```python
from build123d import *

# Parameters (mm, degrees)
SKETCH1_W           = 44
SKETCH1_H           = 44
BOSS_EXTRUDE1_DEPTH = 3
SKETCH2_W           = 21
SKETCH2_H           = 16
BOSS_EXTRUDE2_DEPTH = 12
SKETCH3_W           = 15
SKETCH3_H           = 10
CUT_EXTRUDE1_DEPTH  = 12
CUT_EXTRUDE2_REACH  = 66.008
FILLET1_R           = 3.175


with BuildPart() as part:
    # Sketch1 → Boss-Extrude1 (new body)
    with BuildSketch(Plane(origin=(0, 0, 0), x_dir=(1, 0, 0), z_dir=(0, 1, 0))):
        with Locations((22, 22)):
            Rectangle(SKETCH1_W, SKETCH1_H)
    extrude(amount=BOSS_EXTRUDE1_DEPTH)

    # Sketch2 → Boss-Extrude2 (add)
    with BuildSketch(Plane(origin=(0, 3, 0), x_dir=(1, 0, 0), z_dir=(0, 1, 0))):
        with Locations((22, 22)):
            Rectangle(SKETCH2_W, SKETCH2_H)
    extrude(amount=BOSS_EXTRUDE2_DEPTH)

    # Sketch3 → Cut-Extrude1 (cut)
    with BuildSketch(Plane.XZ):
        with Locations((22, -22)):
            Rectangle(SKETCH3_W, SKETCH3_H)
    extrude(amount=-CUT_EXTRUDE1_DEPTH, mode=Mode.SUBTRACT)

    # Sketch4 → Cut-Extrude2 (cut, up to next)
    with BuildSketch(Plane(origin=(0, 15, 0), x_dir=(1, 0, 0), z_dir=(0, 1, 0)), mode=Mode.PRIVATE) as cut_extrude2_sk1:
        with BuildLine():
            Line((19.05, 23.2), (24.95, 23.2))
            ThreePointArc((24.95, 23.2), (26.15, 22), (24.95, 20.8))
            Line((24.95, 20.8), (19.05, 20.8))
            ThreePointArc((19.05, 20.8), (17.85, 22), (19.05, 23.2))
        make_face()
    cut_extrude2_tool1 = extrude(cut_extrude2_sk1.sketch, amount=-CUT_EXTRUDE2_REACH, mode=Mode.PRIVATE) & part.part
    add(cut_extrude2_tool1.solids().sort_by_distance((22, 15, -22))[0], mode=Mode.SUBTRACT)

    # Fillet1
    fillet1_edges = [part.edges().sort_by_distance(p)[0] for p in [
        (0, 1.5, -44),
        (44, 1.5, -44),
        (44, 1.5, 0),
        (0, 1.5, 0),
    ]]
    fillet(fillet1_edges, radius=FILLET1_R)


solid = part.part
```
Build history of the part. All positions in model axes, mm. A direction names the side the tool comes from. Give positions to 0.01 mm unless a question says otherwise; leave off trailing zeros. Loops run counter-clockwise (first coordinate to the right, second up) from the corner with the lowest first, then second, coordinate; pieces in that order, holes last. Notation, with made-up numbers: (-3, 29) - (40, 29) arc R23 cw to (40, 60) - close; hole circle Ø6 at (59, 66). An arc over 180 degrees is marked (long way). Use a Markdown table: item, result.
(1) Band-saw the part on C-C (y = 11). Give the cut face in (x, z).
Taken from the geometry:
| item | result |
|---|---|
| outline | (11.5, -30) - (32.5, -30) - (32.5, -14) - (11.5, -14) - close; hole (14.5, -27) - (29.5, -27) - (29.5, -17) - (14.5, -17) - close |
(2) Wall check: line 1 along Z through (x, y) = (20.5, 12.75); line 2 along Z through (x, y) = (26, 10.5); line 3 along X through (y, z) = (7, -20). Give the ranges that are in metal, low to high.
Taken from the geometry:
| item | result |
|---|---|
| line 1 | -30 to -23.2, -20.8 to -14 |
| line 2 | -30 to -27, -17 to -14 |
| line 3 | 11.5 to 14.5, 29.5 to 32.5 |
(3) Band-saw the part on D-D (y = 1). Give the cut face in (x, z) (3 decimals), and give its area (3 significant figures).
Taken from the geometry:
| item | result |
|---|---|
| outline | (0, -40.825) arc R3.175 ccw to (3.175, -44) - (40.825, -44) arc R3.175 ccw to (44, -40.825) - (44, -3.175) arc R3.175 ccw to (40.825, 0) - (3.175, 0) arc R3.175 ccw to (0, -3.175) - close; hole (14.5, -27) - (29.5, -27) - (29.5, -17) - (14.5, -17) - close |
| area | 1,780 mm2 |
(4) Band-saw the part on A-A (z = -22). Give the cut face in (x, y), and give its area (3 significant figures).
Taken from the geometry:
| item | result |
|---|---|
| outline | (0, 0) - (14.5, 0) - (14.5, 12) - (17.85, 12) - (17.85, 15) - (11.5, 15) - (11.5, 3) - (0, 3) - close; (26.15, 12) - (29.5, 12) - (29.5, 0) - (44, 0) - (44, 3) - (32.5, 3) - (32.5, 15) - (26.15, 15) - close |
| area | 179 mm2 |
(5) Band-saw the part on B-B (x = 13.5). Give the cut face in (y, z), and give its area (3 significant figures).
Taken from the geometry:
| item | result |
|---|---|
| outline | (0, -44) - (3, -44) - (3, -30) - (15, -30) - (15, -14) - (3, -14) - (3, 0) - (0, 0) - close |
| area | 324 mm2 |
(6) Which spindle directions (+Z, -Z, +X, -X, +Y, -Y) get a long thin tool onto all of the face, cutting with end or side? Do faces 1 (the face through (22, 9, -30)), 2 (the face through (32.5, 9, -22)), 3 (the face through (29.5, 6, -22)). Say none if no direction does.
Taken from the geometry:
| item | result |
|---|---|
| face 1 | -Z, +X, -X, +Y |
| face 2 | +Z, -Z, +X, +Y |
| face 3 | -Y |
(7) Drop flat-ended pins along their axis: pin 1 Ø6 at (x, y) = (25.5, 9) entering from -Z; pin 2 Ø3.5 at (y, z) = (8, -24.5) entering from +X; pin 3 Ø3.5 at (y, z) = (11.5, -22) entering from -X. Give the stop position or say it passes through.
Taken from the geometry:
| item | result |
|---|---|
| pin 1 | z = -30 |
| pin 2 | x = 32.5 |
| pin 3 | x = 11.5 |
